```python
from build123d import *

# Parameters (mm, degrees)
CUT_EXTRUDE1_DEPTH = 25.4


with BuildPart() as part:
    # Sketch1 → Revolve1 (revolve)
    with BuildSketch(Plane.XY):
        with BuildLine():
            Line((-50, 94.429578452), (-43.950074951, 74.146502495))
            add(Edge.make_bspline(
                [(-43.950074951, 74.146502495), (-30.324787154, 69.527502201), (-7.935332232, 64.635999311), (43.950074951, 74.146502495)],
                knots=[0, 0, 0, 0, 1, 1, 1, 1], degree=3))
            Line((43.950074951, 74.146502495), (50, 94.429578452))
            Line((50, 94.429578452), (52.434031632, 93.703568799))
            Line((52.434031632, 93.703568799), (45.843039456, 71.606502495))
            add(Edge.make_bspline(
                [(-5.291699224, 59.717748904), (20.861844129, 60.268983178), (45.843039456, 71.606502495)],
                knots=[0.463836412, 0.463836412, 0.463836412, 1, 1, 1], degree=2))
            Line((-5.291699224, 59.717748904), (-5.291699224, 40))
            Line((-5.291699224, 40), (-7.524484902, 9))
            Line((-7.524484902, 9), (-7.524484902, 59.790811734))
            add(Edge.make_bspline(
                [(-45.843039456, 71.606502495), (-27.071768847, 58.162400144), (-31.463870641, 60.513484529), (-7.524484902, 59.790811734)],
                knots=[0, 0, 0, 0, 0.44581559, 0.44581559, 0.44581559, 0.44581559], degree=3))
            Line((-45.843039456, 71.606502495), (-52.434031632, 93.703568799))
            Line((-52.434031632, 93.703568799), (-50, 94.429578452))
        make_face()
    revolve(axis=Axis((-165.294689037, 0, 0), (1, 0, 0)))

    # Sketch2 → Cut-Extrude1 (cut)
    with BuildSketch(Plane(origin=(-5.291699224, 0, 0), x_dir=(0, 0, -1), z_dir=(1, 0, 0))):
        Polygon((0, 63.958336037), (-9.083437699, 122.299155441), (9.083437699, 122.299155441), align=None)
        Polygon((31.979168019, 55.389543792), (53.283089919, 110.455894323), (69.016065522, 101.372456624), align=None)
        Polygon((55.389543792, 31.979168019), (101.372456624, 69.016065522), (110.455894323, 53.283089919), align=None)
        Polygon((63.958336037, 0), (122.299155441, 9.083437699), (122.299155441, -9.083437699), align=None)
        Polygon((55.389543792, -31.979168019), (110.455894323, -53.283089919), (101.372456624, -69.016065522), align=None)
        Polygon((31.979168019, -55.389543792), (69.016065522, -101.372456624), (53.283089919, -110.455894323), align=None)
        Polygon((0, -63.958336037), (9.083437699, -122.299155441), (-9.083437699, -122.299155441), align=None)
        Polygon((-31.979168019, -55.389543792), (-53.283089919, -110.455894323), (-69.016065522, -101.372456624), align=None)
        Polygon((-55.389543792, -31.979168019), (-101.372456624, -69.016065522), (-110.455894323, -53.283089919), align=None)
        Polygon((-63.958336037, 0), (-122.299155441, -9.083437699), (-122.299155441, 9.083437699), align=None)
        Polygon((-55.389543792, 31.979168019), (-110.455894323, 53.283089919), (-101.372456624, 69.016065522), align=None)
        Polygon((-31.979168019, 55.389543792), (-69.016065522, 101.372456624), (-53.283089919, 110.455894323), align=None)
    extrude(amount=-CUT_EXTRUDE1_DEPTH, mode=Mode.SUBTRACT)


solid = part.part
```
Model file for the job. Use its own axes, mm. Coordinates: 2 decimals unless noted, no trailing zeros. Answer as a JSON object with one key per item and string values. Group by question number.
(1) Probe line 1 along Y through (x, z) = (-24.5, -44); line 2 along Z through (x, y) = (-23.5, 27.5); line 3 along Z through (x, y) = (-15, -15). List the from-to ranges inside material, lowest first.
(2) Flat gauge pins, fed straight in: pin 1 (8 mm diameter, centred on y = -25, z = 24, fed in from -X); pin 2 (4.5 mm diameter, centred on y = -58.5, z = 34.5, fed in from +X); pin 3 (3.5 mm diameter, centred on y = 33.5, z = -57.5, fed in from -X); pin 4 (2 mm diameter, centred on y = -70, z = -63, fed in from -X). Where does each tip first touch, or does it go through?
(3) Two-plate mould, pull along X, no slides. Class faces 1 (the face through (46.163, -9.461, 72.061)), 2 (the face through (-46.255, -72.918, 3.209)), 3 (the face through (-17.814, 33.66, 57.476)): released by +X, released by -X, zero draft, split by the parting line, or undercut.
Geometry says:
{
 "1": {"line 1": "y = -54.04 to -41.13, 41.13 to 54.04", "line 2": "z = -63.9 to -53.51, 53.51 to 63.9", "line 3": "z = -67.23 to -58.04, 58.04 to 67.23"},
 "2": {"pin 1": "stops at x = -7.52", "pin 2": "stops at x = 42.56", "pin 3": "stops at x = -41.23", "pin 4": "stops at x = -52.43"},
 "3": {"face 1": "released by +X", "face 2": "released by -X", "face 3": "undercut"}
}
